Input: dimensioned drawing with shaded views. Units: mm. Origin: part minimum x, y, z. A direction names the side the tool comes from. Round coordinates to 2 decimals unless told otherwise and drop trailing zeros. Loops run counter-clockwise (first coordinate to the right, second up) from the corner with the lowest first, then second, coordinate; pieces in that order, holes last. Notation, with made-up numbers: (-39, 46.5) - (-17, 46.5) arc R25 cw to (-17, 58.5) - close; hole circle Ø2 at (76, 27). An arc over 180 degrees is marked (long way). Use CSV: the item, a comma, the result in double quotes. Start each with the question number.
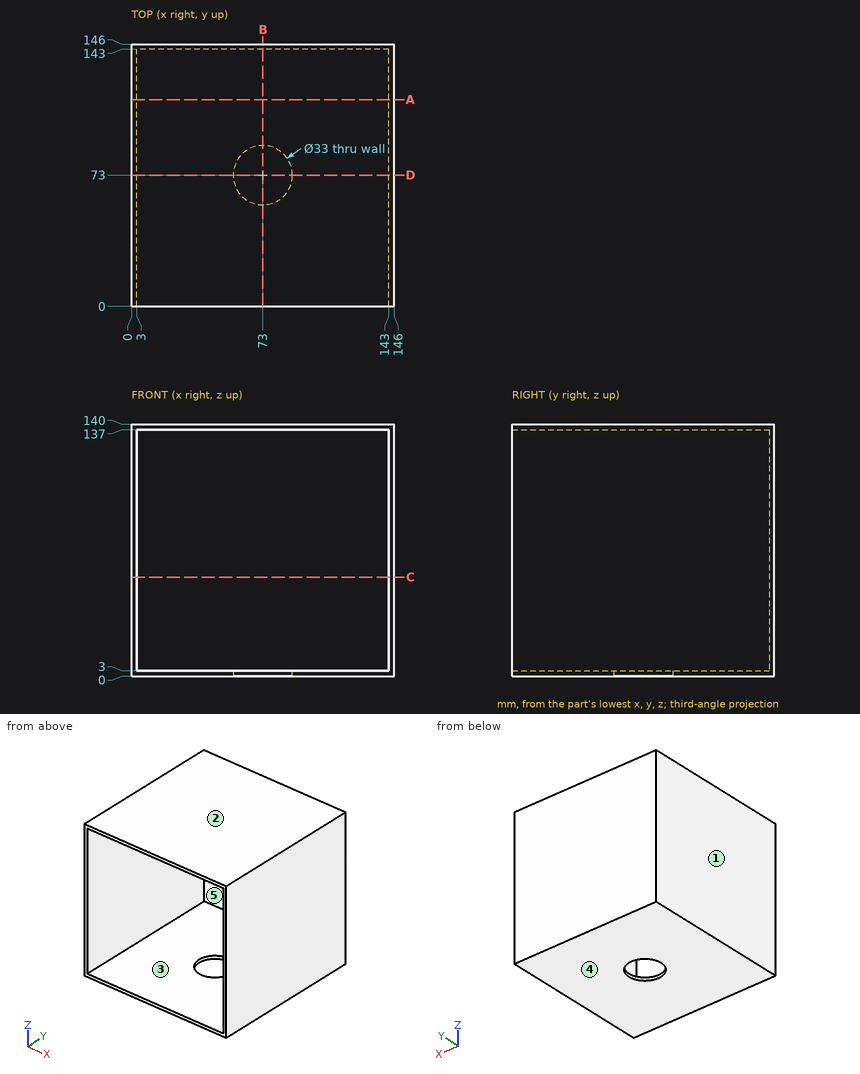
1. Section query C-C on z = 55. Return the cut outline in (x, y), and give its area (3 significant figures).
2. Mould query, pull axis X, two halves, no side actions, for the marked faces 1, 2 and 3. Classes: +X half, -X half, draft (parallel to the pull), parting line (faces both ways), or undercut.
3. Section query B-B on x = 73. Return the cut outline in (y, z), and give its area (3 significant figures).
4. Line query: line 1 along Z through (x, y) = (122.5, 16.5); line 2 along X through (y, z) = (42, 18.5); line 3 along Y through (x, z) = (73, 2). Output: solid intervals per line, ascending.
5. Section query D-D on y = 73. Return the cut outline in (x, z).
6. Section query A-A on y = 115. Return the cut outline in (x, z).
7. Contact query for a flat-ended pin moving along its axis: P1, Ø4, axis at x = 35.5, z = 46.5, coming from the -Y side. Output: stop coordinate, or through.
8. Reachability of the marked faces 4 and 5 from +Z, -Z, +X, -X, +Y, -Y: full face, straight path, thin tool, end or side. Return the list, or none.
Values:
1,outline,"(0, 0) - (3, 0) - (3, 143) - (143, 143) - (143, 0) - (146, 0) - (146, 146) - (0, 146) - close"
1,area,"1,300 mm^2"
2,face 1,"-X half"
2,face 2,"draft"
2,face 3,"undercut"
3,outline,"(0, 0) - (56.5, 0) - (56.5, 3) - (0, 3) - close; (0, 137) - (143, 137) - (143, 3) - (89.5, 3) - (89.5, 0) - (146, 0) - (146, 140) - (0, 140) - close"
3,area,"1,180 mm^2"
4,line 1,"z = 0 to 3, 137 to 140"
4,line 2,"x = 0 to 3, 143 to 146"
4,line 3,"y = 0 to 56.5, 89.5 to 146"
5,outline,"(0, 0) - (56.5, 0) - (56.5, 3) - (3, 3) - (3, 137) - (143, 137) - (143, 3) - (89.5, 3) - (89.5, 0) - (146, 0) - (146, 140) - (0, 140) - close"
6,outline,"(0, 0) - (146, 0) - (146, 140) - (0, 140) - close; hole (3, 3) - (143, 3) - (143, 137) - (3, 137) - close"
7,P1,"stops at y = 143"
8,face 4,"-Z, +X, -X, +Y, -Y"
8,face 5,"-Y"
